Design review of the part shown in the three views and the two pictorial views. Dimensions are in mm from the part's minimum x, y and z. A direction names the side the tool comes from. Coordinates: 2 decimals unless noted, no trailing zeros. Loops run counter-clockwise (first coordinate to the right, second up) from the corner with the lowest first, then second, coordinate; pieces in that order, holes last. Notation, with made-up numbers: M -38,78.5 L 19,78.5 A24 cw 19,113.5 Z; hole C -7,27 d10. An arc over 180 degrees is marked long. Answer as a JSON object with one key per item and string values. Group by question number.
Item 1: Wall thickness on L1, parallel to Z at x = 3, y = 4.5; L2, parallel to X at y = 13.5, z = 8; L3, parallel to Y at x = 6.75, z = 1.25: over which ranges is each line inside the solid? List them lowest first. Write a range as from..to.
Item 2: Add section D-D (x = 7). State the section outline as (y, z) points, then the cut area to 3 significant figures.
Item 3: Add section B-B (z = 8.25). State the section outline as (x, y) points, then the cut area to 3 significant figures.
Item 4: Insertion check: pin 1 (1.9 mm diameter, centred on x = 7, y = 13.5, fed in from -Z); pin 2 (1.9 mm diameter, centred on x = 5.5, y = 13, fed in from +Z); pin 3 (1.5 mm diameter, centred on y = 7.5, z = 8.5, fed in from +X). Each pin has a flat end and moves straight along its axis. Give the tip position at first contact, or say it passes through.
Item 5: Tool access review of the marked faces 1, 2, 3 and 4: name each direction out of +Z, -Z, +X, -X, +Y, -Y from which nothing blocks a thin tool from reaching the whole face with its end or side.
Item 6: Add section A-A (x = 5.4). State the section outline as (y, z) points.
Item 7: Mouldability with a two-part tool opening along Z and no side actions: class the marked faces 5, 6, 7 and 8 as +Z half, -Z half, draft (parallel to the pull), parting line (faces both ways), or undercut.
Item 8: Add section C-C (y = 8). State the section outline as (x, z) points.
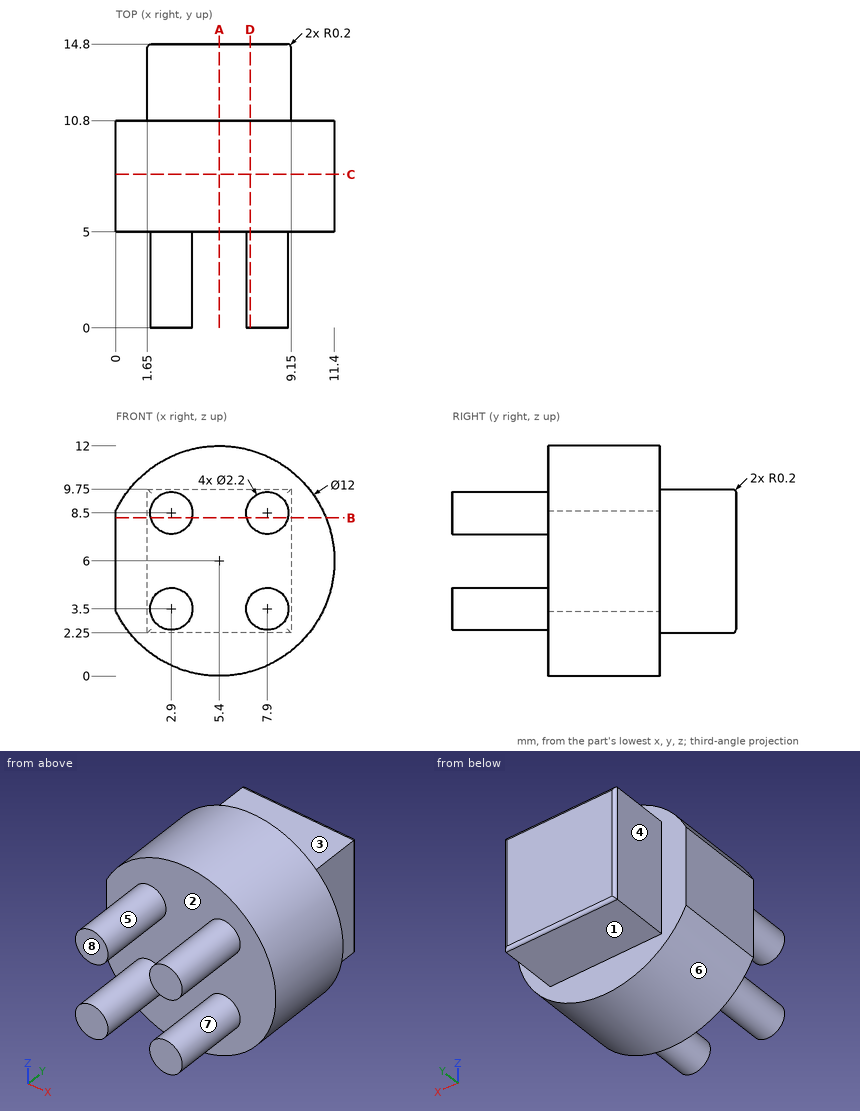
From the geometry:
{
 "1": {"L1": "z = 2.4..4.6, 7.4..9.6", "L2": "x = 1.65..9.15", "L3": "y = 5..10.8"},
 "2": {"outline": "M 0,2.87 L 5,2.87 L 5,0.22 L 10.8,0.22 L 10.8,2.25 L 14.6,2.25 A0.2 ccw 14.8,2.45 L 14.8,9.55 A0.2 ccw 14.6,9.75 L 10.8,9.75 L 10.8,11.78 L 5,11.78 L 5,9.13 L 0,9.13 L 0,7.87 L 5,7.87 L 5,4.13 L 0,4.13 Z", "area": "110 mm²"},
 "3": {"outline": "M 0,5 L 1.83,5 L 1.83,0 L 3.97,0 L 3.97,5 L 6.83,5 L 6.83,0 L 8.97,0 L 8.97,5 L 10.96,5 L 10.96,10.8 L 9.15,10.8 L 9.15,14.6 A0.2 ccw 8.95,14.8 L 1.85,14.8 A0.2 ccw 1.65,14.6 L 1.65,10.8 L 0,10.8 Z", "area": "115 mm²"},
 "4": {"pin 1": "stops at z = 2.25", "pin 2": "stops at z = 9.75", "pin 3": "stops at x = 11.14"},
 "5": {"face 1": "-Z, +X, -X, +Y", "face 2": "-Y", "face 3": "+Z, +X, -X, +Y", "face 4": "+Z, -Z, -X, +Y"},
 "6": {"outline": "M 5,0 L 10.8,0 L 10.8,2.25 L 14.6,2.25 A0.2 ccw 14.8,2.45 L 14.8,9.55 A0.2 ccw 14.6,9.75 L 10.8,9.75 L 10.8,12 L 5,12 Z"},
 "7": {"face 5": "undercut", "face 6": "parting line", "face 7": "undercut", "face 8": "draft"},
 "8": {"outline": "M 0,3.38 A6 ccw long 0,8.62 Z"}
}
